Could you check a few things on this drawing? It's one solid part, dimensions in mm from its lowest x, y, z. Round coordinates to 2 decimals unless told otherwise and drop trailing zeros. Loops run counter-clockwise (first coordinate to the right, second up) from the corner with the lowest first, then second, coordinate; pieces in that order, holes last. Notation, with made-up numbers: M 78,72 L 86,72 A26 ccw 86,102 Z; hole C 0.25,55 d6. An arc over 180 degrees is marked long. Return JSON: item names as keys, results as strings.
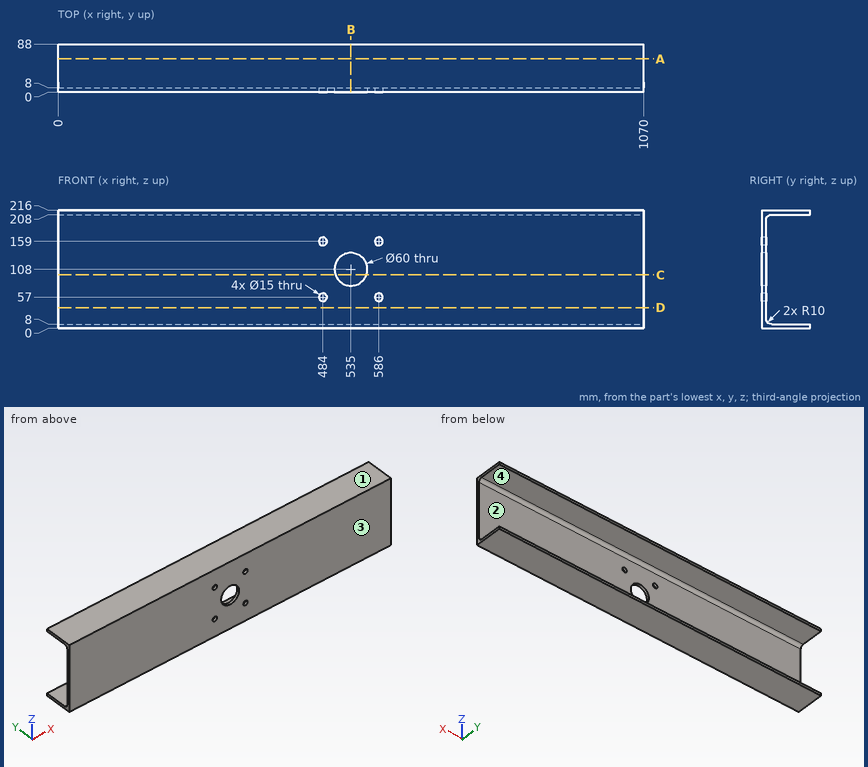
Q1. If I drill on line 1 along X through (y, z) = (2.25, 159); line 2 along Z through (x, y) = (586, 2.75); line 3 along Z through (x, y) = (535, 6.25), over which ranges is the centre line in solid material (lowest first)?
Results:
{"line 1": "x = 0 to 476.5, 491.5 to 578.5, 593.5 to 1070", "line 2": "z = 0 to 49.5, 64.5 to 151.5, 166.5 to 216", "line 3": "z = 0 to 78, 138 to 216"}
Q2. Suppose I cut it at D-D, the plane z = 38. Please give me the cut outline in (x, y), plus the area to 3 significant figures.
Results:
{"outline": "M 0,0 L 1070,0 L 1070,8 L 0,8 Z", "area": "8,560 mm2"}
Q3. Suppose I cut it at A-A, the plane y = 61. Please give me the cut outline in (x, z).
Results:
{"outline": "M 0,0 L 1070,0 L 1070,8 L 0,8 Z; M 0,208 L 1070,208 L 1070,216 L 0,216 Z"}
Q4. I'm going to push a flat-ended pin straight in: pin 1 Ø8 at (x, z) = (812, 58.5) entering from +Y. Where does the tip first touch, or does it pass through?
Results:
{"pin 1": "stops at y = 8"}
Q5. Suppose I cut it at B-B, the plane x = 535. Please give me the cut outline in (y, z), plus the area to 3 significant figures.
Results:
{"outline": "M 0,0 L 88,0 L 88,8 L 18,8 A10 cw 8,18 L 8,78 L 0,78 Z; M 0,138 L 8,138 L 8,198 A10 cw 18,208 L 88,208 L 88,216 L 0,216 Z", "area": "2,570 mm2"}
Q6. Thinking about a two-plate mould opening in Z: for the marked faces 1, 2, 3 and 4, which applies, pulls with the +Z half, pulls with the -Z half, needs draft (parallel to the pull), parting line crosses it, or undercut?
Results:
{"face 1": "pulls with the +Z half", "face 2": "undercut", "face 3": "needs draft", "face 4": "undercut"}
Q7. Suppose I cut it at C-C, the plane z = 98. Please give me the cut outline in (x, y), plus the area to 3 significant figures.
Results:
{"outline": "M 0,0 L 506.72,0 L 506.72,8 L 0,8 Z; M 563.28,0 L 1070,0 L 1070,8 L 563.28,8 Z", "area": "8,110 mm2"}
